Here's how the part is built. I have some questions about the finished solid (model axes, mm). Face numbers are marked on the shaded views. Round coordinates to 2 decimals unless told otherwise and drop trailing zeros. Loops run counter-clockwise (first coordinate to the right, second up) from the corner with the lowest first, then second, coordinate; pieces in that order, holes last. Notation, with made-up numbers: M -7.75,83.25 L 7.25,83.25 A21 ccw 7.25,89.25 Z; hole C -17.5,59.5 d9. An arc over 180 degrees is marked long. Use a Markdown table: item, result.
```python
from build123d import *

# Parameters (mm, degrees)
SKETCH_1_R          = 2.75
EXTRUDE_1_DEPTH     = 3
FILLET_1_R          = 0.5
CUT_EXTRUDE_1_DEPTH = 2
SKETCH_3_R          = 1.5
EXTRUDE_2_DEPTH     = 18
CHAMFER_1_SIZE      = 0.2
FILLET_2_R          = 0.2


with BuildPart() as part:
    # 草图1 → 凸台-拉伸1 (new body)
    with BuildSketch(Plane.XY):
        Circle(SKETCH_1_R)
    extrude(amount=EXTRUDE_1_DEPTH)

    # 圆角1
    fillet_1_edges = [part.edges().sort_by_distance(p)[0] for p in [
        (-2.75, 0, 3),
    ]]
    fillet(fillet_1_edges, radius=FILLET_1_R)

    # 草图2 → 切除-拉伸1 (cut)
    with BuildSketch(Plane.XY.offset(3)):
        Polygon((1.558845727, 0), (0.779422863, 1.35), (-0.779422863, 1.35), (-1.558845727, 0), (-0.779422863, -1.35), (0.779422863, -1.35), align=None)
    extrude(amount=-CUT_EXTRUDE_1_DEPTH, mode=Mode.SUBTRACT)

    # 草图3 → 凸台-拉伸2 (add)
    with BuildSketch(Plane(origin=(0, 0, 0), x_dir=(-1, 0, 0), z_dir=(0, 0, -1))):
        Circle(SKETCH_3_R)
    extrude(amount=EXTRUDE_2_DEPTH)

    # 倒角1
    chamfer_1_edges = [part.edges().sort_by_distance(p)[0] for p in [
        (1.5, 0, -18),
    ]]
    chamfer(chamfer_1_edges, length=CHAMFER_1_SIZE)

    # 圆角2
    fillet_2_edges = [part.edges().sort_by_distance(p)[0] for p in [
        (-2.75, 0, 0),
    ]]
    fillet(fillet_2_edges, radius=FILLET_2_R)


solid = part.part
```
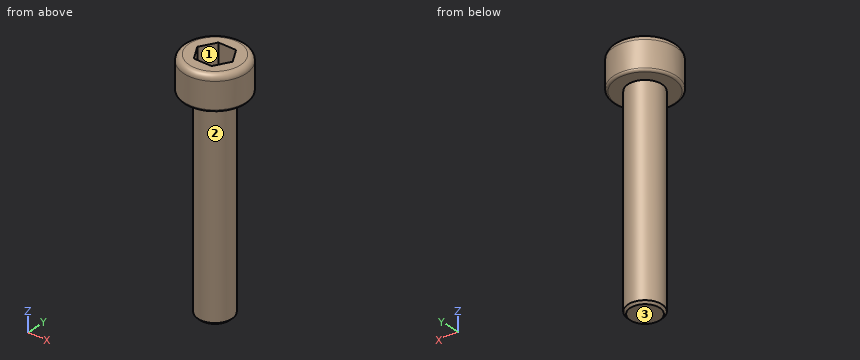
Q1. We'd pull the mould along Y, two halves only. Please class the marked faces 1, 2 and 3: pulls with the +Y half, pulls with the -Y half, needs draft (parallel to the pull), parting line crosses it, or undercut.
Return value:
| item | result |
|---|---|
| face 1 | undercut |
| face 2 | parting line crosses it |
| face 3 | needs draft |
Q2. Will these pins go through, and if not, where does the flat tip stop? P1, Ø3, axis at x = 0.5, z = -10.5, coming from the +Y side; P2, Ø2, axis at x = 2, z = -15, coming from the +Y side; P3, Ø0.8, axis at x = -0.5, y = 0.5, coming from the +Z side.
Return value:
| item | result |
|---|---|
| P1 | stops at y = 1.5 |
| P2 | stops at y = 1.12 |
| P3 | stops at z = 1 |
Q3. Imagine slicing it at B-B, the plane x = 0. Please give me the cut outline in (y, z), then the cut area to 3 significant figures.
Return value:
| item | result |
|---|---|
| outline | M -2.75,0.2 A0.2 ccw -2.55,0 L -1.5,0 L -1.5,-17.8 L -1.3,-18 L 1.3,-18 L 1.5,-17.8 L 1.5,0 L 2.55,0 A0.2 ccw 2.75,0.2 L 2.75,2.5 A0.5 ccw 2.25,3 L 1.35,3 L 1.35,1 L -1.35,1 L -1.35,3 L -2.25,3 A0.5 ccw -2.75,2.5 Z |
| area | 64.9 mm^2 |
Q4. Imagine slicing it at A-A, the plane z = 1.5. Please give me the cut outline in (x, y), then the cut area to 3 significant figures.
Return value:
| item | result |
|---|---|
| outline | C 0,0 d5.5; hole M -1.56,0 L -0.78,-1.35 L 0.78,-1.35 L 1.56,0 L 0.78,1.35 L -0.78,1.35 Z |
| area | 17.4 mm^2 |
Q5. I need wall thicknesses on line 1 (X direction, y = -0.05, z = -8.5); line 2 (Z direction, x = -2, y = -0.85); line 3 (Z direction, x = 1.1, y = 0.55). Which ranges of each line are inside material? Lowest first, please. Write a range as from..to.
Return value:
| item | result |
|---|---|
| line 1 | x = -1.5..1.5 |
| line 2 | z = 0..3 |
| line 3 | z = -18..1 |
Q6. Imagine slicing it at C-C, the plane z = -3. Please give me the cut outline in (x, y), then the cut area to 3 significant figures.
Return value:
| item | result |
|---|---|
| outline | C 0,0 d3 |
| area | 7.07 mm^2 |
